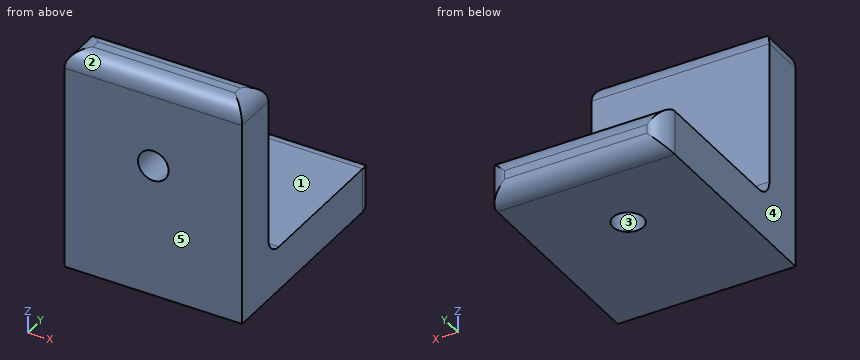
```python
from build123d import *

# Parameters (mm, degrees)
SKETCH1_W                        = 25.4
SKETCH1_H                        = 25.4
BOSS_EXTRUDE1_DEPTH              = 6.35
SKETCH2_W                        = 25.4
SKETCH2_H                        = 31.75
BOSS_EXTRUDE2_DEPTH              = 6.35
FILLET1_R                        = 2.54
F_11_64_0_17188_DIAMETER_HOLE1_D = 4.365752
F_11_64_0_17188_DIAMETER_HOLE2_D = 4.365752


with BuildPart() as part:
    # Sketch1 → Boss-Extrude1 (new body)
    with BuildSketch(Plane(origin=(0, 0, 0), x_dir=(1, 0, 0), z_dir=(0, 1, 0))):
        Rectangle(SKETCH1_W, SKETCH1_H)
    extrude(amount=BOSS_EXTRUDE1_DEPTH)

    # Sketch2 → Boss-Extrude2 (add)
    with BuildSketch(Plane(origin=(0, 0, -12.7), x_dir=(-1, 0, 0), z_dir=(0, 0, -1))):
        with Locations((0, 15.875)):
            Rectangle(SKETCH2_W, SKETCH2_H)
    extrude(amount=BOSS_EXTRUDE2_DEPTH)

    # Fillet1
    fillet1_edges = [part.edges().sort_by_distance(p)[0] for p in [
        (0, 31.75, -12.7),
        (-12.7, 31.75, -15.875),
        (12.7, 31.75, -15.875),
        (0, 6.35, 12.7),
        (0, 31.75, -19.05),
        (0, 0, 12.7),
        (12.7, 3.175, 12.7),
        (-12.7, 3.175, 12.7),
        (0, 6.35, -12.7),
    ]]
    fillet(fillet1_edges, radius=FILLET1_R)

    # 11/64 (0.17188) Diameter Hole1 (through all)
    with Locations(Plane(origin=(0, 6.35, 0), x_dir=(1, 0, 0), z_dir=(0, 1, 0))):
        with Locations((0, 0)):
            Hole(F_11_64_0_17188_DIAMETER_HOLE1_D / 2)

    # 11/64 (0.17188) Diameter Hole2 (through all)
    with Locations(Plane.XY.offset(-12.7)):
        with Locations((0, 19.05)):
            Hole(F_11_64_0_17188_DIAMETER_HOLE2_D / 2)


solid = part.part
```
The model under review builds one solid part; all positions refer to its coordinate system, in mm. Face numbers are marked on the shaded views. A direction names the side the tool comes from. Give positions to 0.01 mm unless a question says otherwise; leave off trailing zeros. Loops run counter-clockwise (first coordinate to the right, second up) from the corner with the lowest first, then second, coordinate; pieces in that order, holes last. Notation, with made-up numbers: (15, -9.5) - (26, -9.5) arc R24 ccw to (26, 26.5) - close; hole circle Ø1 at (34.5, 24). An arc over 180 degrees is marked (long way). Answer as a JSON object with one key per item and string values.
Q1. For the marked faces 1 and 2, list the 3-axis set-ups (+Z, -Z, +X, -X, +Y, -Y) from which the entire face can be reached by the end or side of a thin tool; tool diameter is ignored.
Worked out:
{"face 1": "+Z, +X, -X, +Y", "face 2": "+Z, +X, -X, -Y"}
Q2. Add section A-A on x = 0. State the section outline as (y, z) points, plus the area to 3 significant figures.
Worked out:
{"outline": "(0, -19.05) - (16.87, -19.05) - (16.87, -12.7) - (8.89, -12.7) arc R2.54 cw to (6.35, -10.16) - (6.35, -2.18) - (0, -2.18) - close; (0, 2.18) - (6.35, 2.18) - (6.35, 10.16) arc R2.54 ccw to (3.81, 12.7) - (2.54, 12.7) arc R2.54 ccw to (0, 10.16) - close; (21.23, -19.05) - (29.21, -19.05) arc R2.54 ccw to (31.75, -16.51) - (31.75, -15.24) arc R2.54 ccw to (29.21, -12.7) - (21.23, -12.7) - close", "area": "303 mm^2"}
Q3. Add section D-D on x = -8. State the section outline as (y, z) points, plus the area to 3 significant figures.
Worked out:
{"outline": "(0, -19.05) - (29.21, -19.05) arc R2.54 ccw to (31.75, -16.51) - (31.75, -15.24) arc R2.54 ccw to (29.21, -12.7) - (8.89, -12.7) arc R2.54 cw to (6.35, -10.16) - (6.35, 10.16) arc R2.54 ccw to (3.81, 12.7) - (2.54, 12.7) arc R2.54 ccw to (0, 10.16) - close", "area": "359 mm^2"}
Q4. Add section B-B on z = 0. State the section outline as (x, y) points, plus the area to 3 significant figures.
Worked out:
{"outline": "(-12.7, 0) - (-2.18, 0) - (-2.18, 6.35) - (-12.7, 6.35) - close; (2.18, 0) - (12.7, 0) - (12.7, 6.35) - (2.18, 6.35) - close", "area": "134 mm^2"}
Q5. Mouldability with a two-part tool opening along X and no side actions: class the marked faces 3, 4 and 5 as +X half, -X half, draft (parallel to the pull), parting line (faces both ways), or undercut.
Worked out:
{"face 3": "undercut", "face 4": "-X half", "face 5": "draft"}
Q6. Add section C-C on y = 19.05. State the section outline as (x, z) points.
Worked out:
{"outline": "(-12.7, -19.05) - (-2.18, -19.05) - (-2.18, -12.7) - (-12.7, -12.7) - close; (2.18, -19.05) - (12.7, -19.05) - (12.7, -12.7) - (2.18, -12.7) - close"}
Q7. Insertion check: pin 1 (6 mm diameter, centred on y = 9.5, z = -8.5, fed in from +X); pin 2 (4 mm diameter, centred on x = 5, z = 0.5, fed in from +Y); pin 3 (5 mm diameter, centred on x = 5, y = 22, fed in from +Z). Each pin has a flat end and moves straight along its axis. Give the tip position at first contact, or say it passes through.
Worked out:
{"pin 1": "passes through", "pin 2": "stops at y = 6.35", "pin 3": "stops at z = -12.7"}
Q8. To check wall thickness, follow line 1 along X through (y, z) = (19, -14); line 2 along Z through (x, y) = (0, 2.5); line 3 along Y through (x, z) = (0, -15.75). State the ranges of each line that lie inside material, in increasing order.
Worked out:
{"line 1": "x = -12.7 to -2.18, 2.18 to 12.7", "line 2": "z = -19.05 to -2.18, 2.18 to 12.7", "line 3": "y = 0 to 16.87, 21.23 to 31.75"}
